from build123d import *

# Parameters (mm, degrees)
SKETCH1_W           = 48
SKETCH1_H           = 300
SKETCH1_R           = 7
SKETCH1_R_2         = 2
BOSS_EXTRUDE1_DEPTH = 5
CHAMFER1_SIZE       = 3


with BuildPart() as part:
    # Sketch1 → Boss-Extrude1 (new body)
    with BuildSketch(Plane.XY):
        with Locations((24, -150)):
            Rectangle(SKETCH1_W, SKETCH1_H)
        with Locations((24, -160)):
            Circle(SKETCH1_R, mode=Mode.SUBTRACT)
        with Locations((8, -144)):
            Circle(SKETCH1_R_2, mode=Mode.SUBTRACT)
        with Locations((16, -144)):
            Circle(SKETCH1_R_2, mode=Mode.SUBTRACT)
        with Locations((24, -144)):
            Circle(SKETCH1_R_2, mode=Mode.SUBTRACT)
        with Locations((32, -144)):
            Circle(SKETCH1_R_2, mode=Mode.SUBTRACT)
        with Locations((40, -144)):
            Circle(SKETCH1_R_2, mode=Mode.SUBTRACT)
        with Locations((16, -152)):
            Circle(SKETCH1_R_2, mode=Mode.SUBTRACT)
        with Locations((32, -152)):
            Circle(SKETCH1_R_2, mode=Mode.SUBTRACT)
        with Locations((40, -152)):
            Circle(SKETCH1_R_2, mode=Mode.SUBTRACT)
        with Locations((40, -160)):
            Circle(SKETCH1_R_2, mode=Mode.SUBTRACT)
        with Locations((16, -168)):
            Circle(SKETCH1_R_2, mode=Mode.SUBTRACT)
        with Locations((32, -168)):
            Circle(SKETCH1_R_2, mode=Mode.SUBTRACT)
        with Locations((40, -168)):
            Circle(SKETCH1_R_2, mode=Mode.SUBTRACT)
        with Locations((16, -176)):
            Circle(SKETCH1_R_2, mode=Mode.SUBTRACT)
        with Locations((24, -176)):
            Circle(SKETCH1_R_2, mode=Mode.SUBTRACT)
        with Locations((32, -176)):
            Circle(SKETCH1_R_2, mode=Mode.SUBTRACT)
        with Locations((40, -176)):
            Circle(SKETCH1_R_2, mode=Mode.SUBTRACT)
        with Locations((8, -152)):
            Circle(SKETCH1_R_2, mode=Mode.SUBTRACT)
        with Locations((8, -160)):
            Circle(SKETCH1_R_2, mode=Mode.SUBTRACT)
        with Locations((8, -168)):
            Circle(SKETCH1_R_2, mode=Mode.SUBTRACT)
        with Locations((8, -176)):
            Circle(SKETCH1_R_2, mode=Mode.SUBTRACT)
    extrude(amount=BOSS_EXTRUDE1_DEPTH)

    # Chamfer1
    chamfer1_edges = [part.edges().sort_by_distance(p)[0] for p in [
        (48, 0, 2.5),
        (0, 0, 2.5),
    ]]
    chamfer(chamfer1_edges, length=CHAMFER1_SIZE)


solid = part.part
Could you check a few things on this model? Use its own coordinates, in mm. Give positions to 0.01 mm unless a question says otherwise; leave off trailing zeros. Answer in a Markdown table with one row per item. Add a question column.
Item 1: We'd pull the mould along Y, two halves only. Please class faces 1 (the cylindrical face through (22.483, -166.834, 2.465)), 2 (the flat face through (24, -148, 5)), 3 (the flat face through (24, 0, 2)): pulls with the +Y half, pulls with the -Y half, needs draft (parallel to the pull), parting line crosses it, or undercut.
Item 2: I'm going to push flat-ended pins straight in: P1, Ø3.5, axis at x = 24, y = -144, coming from the -Z side; P2, Ø4.5, axis at x = 16, y = -144, coming from the -Z side. Where does each tip first touch, or does it pass through?
Item 3: Please list where these lines run through material, in increasing order: probe 1 along X at (y, z) = (-152, 3.15); probe 2 along Y at (x, z) = (24, 3.3); probe 3 along Y at (x, z) = (16, 2.35).
Item 4: Imagine slicing it at A-A (z = 2.3). Count the separate pieces of the cut face and the enclosed holes in it, and give its area (3 significant figures).
Result:
| question | item | result |
|---|---|---|
| 1 | face 1 | undercut |
| 1 | face 2 | needs draft |
| 1 | face 3 | pulls with the +Y half |
| 2 | P1 | through |
| 2 | P2 | z = 0 |
| 3 | probe 1 | 0 to 6, 10 to 14, 18 to 30, 34 to 38, 42 to 48 |
| 3 | probe 2 | -300 to -178, -174 to -167, -153 to -146, -142 to 0 |
| 3 | probe 3 | -300 to -178, -174 to -170, -166 to -154, -150 to -146, -142 to 0 |
| 4 | separate pieces | 1 |
| 4 | enclosed holes | 21 |
| 4 | area | 14,000 mm2 |
